Part model, mm, in its own coordinate system. A direction names the side the tool comes from. Round coordinates to 2 decimals unless told otherwise and drop trailing zeros. Write each loop counter-clockwise with the first axis right and the second up, starting at its lowest first coordinate (ties: lowest second). Pieces come first, ordered by that corner, then holes. Notation, with made-up numbers: M -7,44.25 L 10,44.25 A24 ccw 10,57.25 Z; hole C 51,88 d8. An arc over 180 degrees is marked long. Answer as a JSON object with one key per item and string values. Group by question number.
1. Drill centre lines: line 1 (X direction, y = 8.5, z = 8.25); line 2 (Z direction, x = 10.75, y = 6.5); line 3 (Y direction, x = 4.75, z = 9). Where is each one in solid material? Low to high. Write a range as from..to.
2. Band-saw the part on A-A, the plane y = 14.5. Write the cut outline in (x, z), plus the area to 3 significant figures.
3. Drop flat-ended pins along their axis: pin 1 (2 mm diameter, centred on x = 4, z = 11, fed in from -Y); pin 2 (6 mm diameter, centred on x = 10.5, y = 17, fed in from +Z); pin 3 (0.9 mm diameter, centred on x = 2.5, y = 13, fed in from +Z); pin 4 (2.5 mm diameter, centred on x = 8, z = 2.5, fed in from +Y). Give the stop position or say it passes through.
4. Band-saw the part on B-B, the plane z = 9.5. Write the cut outline in (x, y).
5. Which spindle directions (+Z, -Z, +X, -X, +Y, -Y) get a long thin tool onto all of the face, cutting with end or side? Do faces 1 (the face through (4.45, 12, 7)), 2 (the face through (1.75, 19.715, 13.126)), 3 (the face through (5.95, 14, 2)). Say none if no direction does.
6. Band-saw the part on D-D, the plane y = 4.5. Write the cut outline in (x, z).
7. Two-plate mould, pull along X, no slides. Class faces 4 (the face through (13.149, 19.715, 12.874)), 5 (the face through (7, 8, 4)), 6 (the face through (7, 8, 0)): +X half, -X half, draft (parallel to the pull), parting line (faces both ways), or undercut.
8. Band-saw the part on C-C, the plane y = 9. Write the cut outline in (x, z).
from build123d import *

# Parameters (mm, degrees)
SKETCH_2_W          = 12
SKETCH_2_H          = 20
EXTRUDE_1_DEPTH     = 4
EXTRUDE_START       = -4
SKETCH_3_W          = 12
SKETCH_3_H          = 4
EXTRUDE_2_DEPTH     = 27
SKETCH_4_W          = 3
SKETCH_4_H          = 8
EXTRUDE_3_DEPTH     = 7
FILLET_5_R          = 5
CUT_EXTRUDE_2_DEPTH = 36.678984208
FILLET_6_R          = 1


with BuildPart() as part:
    # 草图2 → 凸台-拉伸1 (new body)
    with BuildSketch(Plane.XY):
        with Locations((7.449786368, 9.999747852)):
            Rectangle(SKETCH_2_W, SKETCH_2_H)
        with BuildLine():
            Line((5.949786368, 6.499747852), (5.949786368, 2.999747852))
            ThreePointArc((5.949786368, 2.999747852), (7.449786368, 1.499747852), (8.949786368, 2.999747852))
            Line((8.949786368, 2.999747852), (8.949786368, 6.499747852))
            Line((8.949786368, 6.499747852), (5.949786368, 6.499747852))
        make_face(mode=Mode.SUBTRACT)
        with BuildLine():
            Line((5.949786368, 11.999747852), (8.949786368, 11.999747852))
            Line((8.949786368, 11.999747852), (8.949786368, 16.999747852))
            ThreePointArc((8.949786368, 16.999747852), (7.449786368, 18.499747852), (5.949786368, 16.999747852))
            Line((5.949786368, 16.999747852), (5.949786368, 11.999747852))
        make_face(mode=Mode.SUBTRACT)
    extrude(amount=EXTRUDE_1_DEPTH)

    # 草图3 → 凸台-拉伸2 (add)
    with BuildSketch(Plane.XY.offset(4).offset(EXTRUDE_START)):
        with Locations((7.449786368, 17.999747852)):
            Rectangle(SKETCH_3_W, SKETCH_3_H)
    extrude(amount=EXTRUDE_2_DEPTH)

    # 草图4 → 凸台-拉伸3 (add)
    with BuildSketch(Plane.XY.offset(4)):
        with Locations((2.949786368, 11.999747852)):
            Rectangle(SKETCH_4_W, SKETCH_4_H)
        with Locations((11.949786368, 11.999747852)):
            Rectangle(SKETCH_4_W, SKETCH_4_H)
    extrude(amount=EXTRUDE_3_DEPTH)

    # 圆角5
    fillet_5_edges = [part.edges().sort_by_distance(p)[0] for p in [
        (1.449786368, 17.999747852, 27),
        (13.449786368, 17.999747852, 27),
    ]]
    fillet(fillet_5_edges, radius=FILLET_5_R)

    # 草图8 → 切除-拉伸2 (cut, through all)
    with BuildSketch(Plane.ZY.offset(-1.449786368)):
        Polygon((0, 16.999747852), (6, 19.999747852), (0, 19.999747852), align=None)
    extrude(amount=-CUT_EXTRUDE_2_DEPTH, mode=Mode.SUBTRACT)

    # 圆角6
    fillet_6_edges = [part.edges().sort_by_distance(p)[0] for p in [
        (11.985320274, 15.999747852, 25.535533906),
        (7.449786368, 16.999747852, 0),
        (7.449786368, 19.999747852, 6),
        (1.449786368, 15.999747852, 16.5),
        (13.449786368, 15.999747852, 16.5),
        (7.449786368, 15.999747852, 27),
        (7.449786368, 19.999747852, 27),
        (1.449786368, 19.999747852, 14),
        (13.449786368, 19.999747852, 14),
        (2.914252462, 19.999747852, 25.535533906),
        (11.985320274, 19.999747852, 25.535533906),
        (2.914252462, 15.999747852, 25.535533906),
    ]]
    fillet(fillet_6_edges, radius=FILLET_6_R)


solid = part.part
Worked answers:
{
 "1": {"line 1": "x = 1.45..4.45, 10.45..13.45", "line 2": "z = 0..4", "line 3": "y = 16..20"},
 "2": {"outline": "M 1.45,0 L 5.95,0 L 5.95,4 L 4.45,4 L 4.45,11 L 1.45,11 Z; M 8.95,0 L 13.45,0 L 13.45,11 L 10.45,11 L 10.45,4 L 8.95,4 Z", "area": "78.0 mm^2"},
 "3": {"pin 1": "stops at y = 8", "pin 2": "stops at z = 27", "pin 3": "stops at z = 11", "pin 4": "stops at y = 18.87"},
 "4": {"outline": "M 1.45,8 L 4.45,8 L 4.45,16 L 10.45,16 L 10.45,8 L 13.45,8 L 13.45,19 A1 ccw 12.45,20 L 2.45,20 A1 ccw 1.45,19 Z"},
 "5": {"face 1": "+Z, -Y", "face 2": "+Z, -Z, -X, +Y", "face 3": "+Z, -Z"},
 "6": {"outline": "M 1.45,0 L 5.95,0 L 5.95,4 L 1.45,4 Z; M 8.95,0 L 13.45,0 L 13.45,4 L 8.95,4 Z"},
 "7": {"face 4": "+X half", "face 5": "undercut", "face 6": "draft"},
 "8": {"outline": "M 1.45,0 L 13.45,0 L 13.45,11 L 10.45,11 L 10.45,4 L 4.45,4 L 4.45,11 L 1.45,11 Z"}
}
